Source: CAD feature listing. Evaluate the final solid. Frame: model axes, mm. A direction names the side the tool comes from. Coordinates: 2 decimals unless noted, no trailing zeros. Order: outer loops, then holes, each group sorted by start corner. A loop starts at its lowest first (then second) coordinate and runs counter-clockwise, first axis right, second up.
Item 1: Reachability of faces 4 (the flat face through (-4, 4, 18)), 5 (the flat face through (0, 0, 0)), 6 (the flat face through (-4, 4, 62)) from +Z, -Z, +X, -X, +Y, -Y: full face, straight path, thin tool, end or side. Return the list, or none.
Item 2: Section D-D on z = 32. Return the cut outline in (x, y), then the cut area to 3 significant figures.
Item 3: Contact query for flat-ended pins moving along their axis: P1, Ø2, axis at x = 1.5, z = 37, coming from the +Y side; P2, Ø3, axis at y = 0, z = 76.5, coming from the -X side; P3, Ø3, axis at y = 0, z = 3.5, coming from the -X side. Output: stop coordinate, or through.
Item 4: Section A-A on y = 0. State how many separate pieces and enclosed holes the cut face has, then the cut area to 3 significant figures.
Item 5: Mould query, pull axis Y, two halves, no side actions, for faces 1 (the cylindrical face through (-6, 0, 40)), 2 (the flat face through (0, 0, 80)), 3 (the cylindrical face through (0.055, 0.36, 2.355)). Classes: released by +Y, released by -Y, zero draft, split by the parting line, or undercut.
Item 6: Section B-B on z = 71. Return the cut outline in (x, y).
Item 7: Ray query, line 1 (Z direction, x = -2.75, y = 0); line 2 (Z direction, x = 1.5, y = -5.5); line 3 (Z direction, x = 3.5, y = 0.25). Return the intervals inside material, ascending.
from build123d import *

# Parameters (mm, degrees)
SKETCH1_R           = 3.95
BOSS_EXTRUDE1_DEPTH = 13
SKETCH2_R           = 5
BOSS_EXTRUDE2_DEPTH = 5
SKETCH3_R           = 6
BOSS_EXTRUDE3_DEPTH = 44
SKETCH4_R           = 5
BOSS_EXTRUDE4_DEPTH = 5
SKETCH5_R           = 3.95
BOSS_EXTRUDE5_DEPTH = 13
FILLET1_R           = 1
SKETCH6_R           = 1.2
CUT_EXTRUDE1_DEPTH  = 6.5


with BuildPart() as part:
    # Sketch1 → Boss-Extrude1 (new body)
    with BuildSketch(Plane.XY):
        Circle(SKETCH1_R)
    extrude(amount=BOSS_EXTRUDE1_DEPTH)

    # Sketch2 → Boss-Extrude2 (add)
    with BuildSketch(Plane.XY.offset(13)):
        Circle(SKETCH2_R)
    extrude(amount=BOSS_EXTRUDE2_DEPTH)

    # Sketch3 → Boss-Extrude3 (add)
    with BuildSketch(Plane.XY.offset(18)):
        Circle(SKETCH3_R)
    extrude(amount=BOSS_EXTRUDE3_DEPTH)

    # Sketch4 → Boss-Extrude4 (add)
    with BuildSketch(Plane.XY.offset(62)):
        Circle(SKETCH4_R)
    extrude(amount=BOSS_EXTRUDE4_DEPTH)

    # Sketch5 → Boss-Extrude5 (add)
    with BuildSketch(Plane.XY.offset(67)):
        Circle(SKETCH5_R)
    extrude(amount=BOSS_EXTRUDE5_DEPTH)

    # Fillet1
    fillet1_edges = [part.edges().sort_by_distance(p)[0] for p in [
        (-3.95, 0, 0),
        (-3.95, 0, 80),
    ]]
    fillet(fillet1_edges, radius=FILLET1_R)

    # Sketch6 → Cut-Extrude1 (cut, symmetric)
    with BuildSketch(Plane(origin=(0, 0, 0), x_dir=(0, 0, -1), z_dir=(1, 0, 0))):
        with Locations((-76.5, 0)):
            Circle(SKETCH6_R)
        with Locations((-3.5, 0)):
            Circle(SKETCH6_R)
    extrude(amount=CUT_EXTRUDE1_DEPTH, both=True, mode=Mode.SUBTRACT)


solid = part.part
Answer list:
1. face 4: -Z
1. face 5: -Z, +X, -X, +Y, -Y
1. face 6: +Z
2. outline: circle Ø12 at (0, 0)
2. area: 113 mm2
3. P1: stops at y = 5.98
3. P2: stops at x = -3.95
3. P3: stops at x = -3.95
4. separate pieces: 3
4. enclosed holes: 0
4. area: 795 mm2
5. face 1: split by the parting line
5. face 2: zero draft
5. face 3: undercut
6. outline: circle Ø7.9 at (0, 0)
7. line 1: z = 0 to 2.3, 4.7 to 75.3, 77.7 to 80
7. line 2: z = 18 to 62
7. line 3: z = 0.17 to 2.33, 4.67 to 75.33, 77.67 to 79.83
